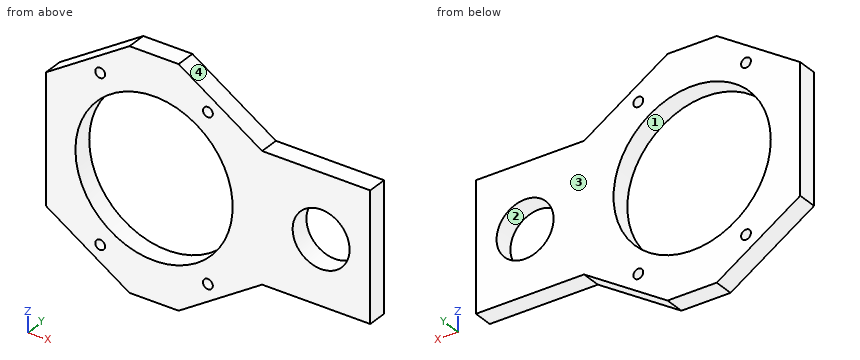
Solid Edge part; units mm, degrees
sketch "Sketch1" plane through (0, 0, 0) normal (0, -1, 0) x (1, 0, 0)
  line L0 (-176.0885, -26.4817) -> (153.9115, -26.4817)
  line L1 (153.9115, -26.4817) -> (153.9115, 213.5183)
  line L2 (-176.0885, 213.5183) -> (153.9115, 213.5183)
  line L3 (-176.0885, -26.4817) -> (-176.0885, 213.5183)
  dimension "D1" = 176.0885
  dimension "D2" = 153.9115
extrude "Protrusion1" add sketch "Sketch1" against normal blind 20
sketch "Sketch2" plane through (3.9115, 20, 48.5183) normal (0, 1, 0) x (-1, 0, 0)
  circle A0 centre (70, 45) radius 80
extrude "Cutout1" cut sketch "Sketch2" against normal through all
sketch "Sketch3" plane through (3.9115, 20, 38.5183) normal (0, 1, 0) x (-1, 0, 0)
  circle A0 centre (-100, 55) radius 29
  dimension "D1" = 100
extrude "Cutout2" cut sketch "Sketch3" against normal through all
sketch "Sketch4" plane through (3.9115, 20, 73.5183) normal (0, 1, 0) x (-1, 0, 0)
  line L0 (180, 85) -> (95, 140)
  line L1 (95, 140) -> (180, 140)
  line L2 (180, 140) -> (180, 85)
  line L3 (-150, 140) -> (-150, 85)
  line L4 (-40, 85) -> (-150, 85)
  line L5 (45, 140) -> (-40, 85)
  line L6 (-150, 140) -> (45, 140)
  dimension "D1" = 150
  dimension "D2" = 150
  dimension "D3" = 95
  dimension "D4" = 180
  dimension "D5" = 40
  dimension "D6" = 150
extrude "Cutout3" cut sketch "Sketch4" against normal through all
hole "Hole_9" at (-11.2875, 20, 9.8711) direction (0, -1, 0) diameter 10 end up to next
hole "Hole1" at (-120.8894, 20, 9.8711) direction (0, -1, 0) diameter 10 end up to next
mirror "Mirror1" about plane through (-73.5885, 5, 93.5183) normal (0, 0, 1) of "Cutout3", "Hole_9", "Hole1"
Can you work these out from the model? Positions are in its coordinate system, mm. Face numbers are marked on the shaded views. Coordinates: 2 decimals unless noted, no trailing zeros. Write each loop counter-clockwise with the first axis right and the second up, starting at its lowest first coordinate (ties: lowest second). Pieces come first, ordered by that corner, then holes. Notation, with made-up numbers: (-1.5, 24) - (33.5, 24) arc R27 cw to (33.5, 49) - close; hole circle Ø9 at (26.5, -13.5). An arc over 180 degrees is marked (long way). Return JSON: item names as keys, results as strings.
Q1. If we section it at B-B (x = -33.5): Please give me the cut outline in (y, z), then the cut area to 3 significant figures.
Computed values:
{"outline": "(0, -21.57) - (20, -21.57) - (20, 20.46) - (0, 20.46) - close; (0, 166.58) - (20, 166.58) - (20, 208.61) - (0, 208.61) - close", "area": "1,680 mm2"}
Q2. If we section it at C-C (y = 15): Please give me the cut outline in (x, z), then the cut area to 3 significant figures.
Computed values:
{"outline": "(-176.09, 28.52) - (-91.09, -26.48) - (-41.09, -26.48) - (43.91, 28.52) - (153.91, 28.52) - (153.91, 158.52) - (43.91, 158.52) - (-41.09, 213.52) - (-91.09, 213.52) - (-176.09, 158.52) - close; hole circle Ø160 at (-66.09, 93.52); hole circle Ø10 at (-120.89, 9.87); hole circle Ø10 at (-120.89, 177.17); hole circle Ø10 at (-11.29, 9.87); hole circle Ø10 at (-11.29, 177.17); hole circle Ø58 at (103.91, 93.52)", "area": "34,700 mm2"}
Q3. I'm going to push flat-ended pins straight in: pin 1 Ø6 at (x, z) = (-120.89, 177.17) entering from +Y; pin 2 Ø2 at (x, y) = (105, 11.5) entering from -Z. Where does each tip first touch, or does it pass through?
Computed values:
{"pin 1": "passes through", "pin 2": "stops at z = 28.52"}
Q4. Thinking about a two-plate mould opening in Z: for the marked faces 1, 2, 3 and 4, which applies, +Z half, -Z half, draft (parallel to the pull), parting line (faces both ways), or undercut?
Computed values:
{"face 1": "undercut", "face 2": "undercut", "face 3": "draft", "face 4": "+Z half"}
Q5. If we section it at D-D (z = 191.5): Please give me the cut outline in (x, y).
Computed values:
{"outline": "(-125.12, 0) - (-7.06, 0) - (-7.06, 20) - (-125.12, 20) - close"}
Q6. Please list where these lines run through material, in increasing order: L1, parallel to X at y = 4.75, z = 94.5; L2, parallel to Z at x = -63, y = 6.5; L3, parallel to X at y = 15.25, z = 6.5. Write a range as from..to.
Computed values:
{"L1": "x = -176.09..-146.08, 13.91..74.93, 132.89..153.91", "L2": "z = -26.48..13.58, 173.46..213.52", "L3": "x = -142.06..-124.58, -117.2..-14.98, -7.59..9.88"}
Q7. If we section it at A-A (z = 145): Please give me the cut outline in (x, y).
Computed values:
{"outline": "(-176.09, 0) - (-127.32, 0) - (-127.32, 20) - (-176.09, 20) - close; (-4.85, 0) - (153.91, 0) - (153.91, 20) - (-4.85, 20) - close"}
